Read the model definition and answer for the solid it produces. Units are mm, in the model's axes. Round coordinates to 2 decimals unless told otherwise and drop trailing zeros. Loops run counter-clockwise (first coordinate to the right, second up) from the corner with the lowest first, then second, coordinate; pieces in that order, holes last. Notation, with made-up numbers: M 15,84 L 67,84 A34 ccw 67,116 Z; hole C 48.25,29 d10. An arc over 180 degrees is marked long. Write each question's results on one line, items separated by ' | '.
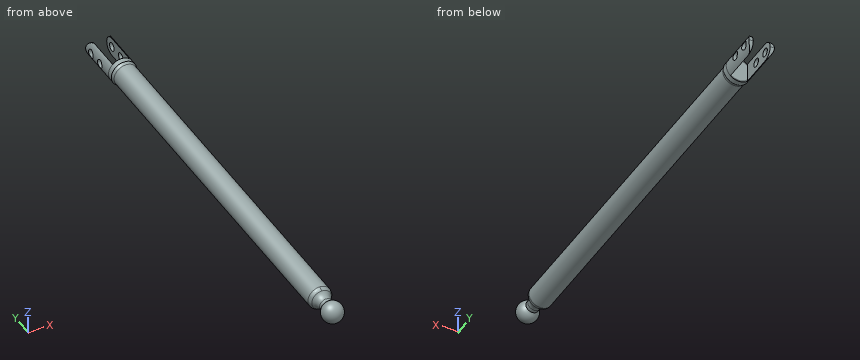
from build123d import *

# Parameters (mm, degrees)
ESBO_O2_R                         = 6
RESSALTO_EXTRUS_O1_DEPTH          = 20
ESBO_O3_R                         = 11
RESSALTO_EXTRUS_O2_DEPTH          = 350
FILETE1_R                         = 10
FILETE2_R                         = 5
RESSALTO_EXTRUS_O3_DEPTH          = 40
RESSALTO_EXTRUS_O4_START          = -5
ESBO_O7_R                         = 12
RESSALTO_EXTRUS_O4_DEPTH          = 5
FILETE3_R                         = 5
CORTE_EXTRUS_O1_DEPTH             = 17.5
CORTE_EXTRUS_O2_REACH             = 412.663
ESBO_O10_R                        = 4
CORTE_EXTRUS_O2_DIRECTION_2_REACH = 412.663


with BuildPart() as part:
    # Esboço1 → Revolução1 (revolve)
    with BuildSketch(Plane.XY):
        with BuildLine():
            Line((-10, 0), (10, 0))
            ThreePointArc((10, 0), (0, 10), (-10, 0))
        make_face()
    revolve(axis=Axis((-10, 0, 0), (1, 0, 0)))

    # Esboço2 → Ressalto-extrusão1 (add)
    with BuildSketch(Plane(origin=(0, 0, 0), x_dir=(1, 0, 0), z_dir=(0, 1, 0))):
        with Locations(Location((0, 0, 0), (0, 0, 90))):
            Circle(ESBO_O2_R)
    extrude(amount=RESSALTO_EXTRUS_O1_DEPTH)

    # Esboço3 → Ressalto-extrusão2 (add)
    with BuildSketch(Plane(origin=(0, 20, 0), x_dir=(1, 0, 0), z_dir=(0, 1, 0))):
        with Locations(Location((0, 0, 0), (0, 0, 270))):
            Circle(ESBO_O3_R)
    extrude(amount=RESSALTO_EXTRUS_O2_DEPTH)

    # Filete1
    # the kernel refuses this fillet: 10 mm, written as the material it adds along each edge
    with BuildSketch(Plane(origin=(0, 20, 0), x_dir=(0, 0, -1), z_dir=(1, 0, 0))) as filete1_piece_1:
        with BuildLine():
            CenterArc((16, -8.660254038), FILETE1_R, 120, 60)
            Line((6, -8.660254038), (5.8, -8.660254038))
            Line((5.8, -8.660254038), (5.8, 0))
            Line((5.8, 0), (6, 0.2))
            ThreePointArc((6, 0.2), (8.5, 0.2), (10.9, 0.173205081))
            Line((10.9, 0.173205081), (11, 0))
        make_face()
    revolve(axis=Axis((0, 20, 0), (0, 1, 0)))

    # Filete2
    filete2_edges = [part.edges().sort_by_distance(p)[0] for p in [
        (11, 20, 0),
    ]]
    fillet(filete2_edges, radius=FILETE2_R)

    # Esboço5 → Ressalto-extrusão3 (add)
    with BuildSketch(Plane(origin=(0, 370, 0), x_dir=(1, 0, 0), z_dir=(0, 1, 0))):
        with BuildLine():
            Line((-8, -8.94427191), (-8, 8.94427191))
            ThreePointArc((-8, 8.94427191), (-12, 0), (-8, -8.94427191))
        make_face()
        with BuildLine():
            Line((8, -8.94427191), (8, 8.94427191))
            ThreePointArc((8, 8.94427191), (12, 0), (8, -8.94427191))
        make_face()
    extrude(amount=RESSALTO_EXTRUS_O3_DEPTH)

    # Esboço7 → Ressalto-extrusão4 (add)
    with BuildSketch(Plane(origin=(0, 370, 0), x_dir=(1, 0, 0), z_dir=(0, 1, 0)).offset(RESSALTO_EXTRUS_O4_START)):
        with Locations(Location((0, 0, 0), (0, 0, 131.810314896))):
            Circle(ESBO_O7_R)
    extrude(amount=RESSALTO_EXTRUS_O4_DEPTH)

    # Filete3
    # the kernel refuses this fillet: 5 mm, written as the material it adds along each edge
    with BuildSketch(Plane(origin=(0, 365, 0), x_dir=(0, 0, 1), z_dir=(1, 0, 0))) as filete3_piece_1:
        with BuildLine():
            CenterArc((16, 3), FILETE3_R, 180, 36.869897646)
            Line((12, 0), (11.92, -0.06))
            ThreePointArc((11.92, -0.06), (11.5, -0.1), (11, -0.1))
            Line((11, -0.1), (10.9, 0))
            Line((10.9, 0), (10.9, 3))
            Line((10.9, 3), (11, 3))
        make_face()
    revolve(axis=Axis((0, 365, 0), (0, -1, 0)))

    # Esboço9 → Corte-extrusão1 (cut, symmetric)
    with BuildSketch(Plane(origin=(0, 0, 0), x_dir=(0, 0, -1), z_dir=(1, 0, 0))):
        with BuildLine():
            Line((-8.94427191, 410), (-8.94427191, 401.05572809))
            ThreePointArc((-8.94427191, 401.05572809), (-6.32455539, 407.38028334), (-1.98e-07, 410))
            Line((-1.98e-07, 410), (-8.94427191, 410))
        make_face()
        with BuildLine():
            Line((8.94427191, 410), (-1.98e-07, 410))
            ThreePointArc((-1.98e-07, 410), (6.32455525, 407.38028348), (8.94427191, 401.05572809))
            Line((8.94427191, 401.05572809), (8.94427191, 410))
        make_face()
    extrude(amount=CORTE_EXTRUS_O1_DEPTH, both=True, mode=Mode.SUBTRACT)

    # Esboço10 → Corte-extrusão2 (cut, up to next)
    with BuildSketch(Plane.ZY.offset(-8), mode=Mode.PRIVATE) as corte_extrus_o2_sk1:
        with Locations((0, 385.527864045)):
            Circle(ESBO_O10_R)
    corte_extrus_o2_tool1 = extrude(corte_extrus_o2_sk1.sketch, amount=-CORTE_EXTRUS_O2_REACH, mode=Mode.PRIVATE) & part.part
    # Esboço10 → Corte-extrusão2 (cut, up to next)
    with BuildSketch(Plane.ZY.offset(-8), mode=Mode.PRIVATE) as corte_extrus_o2_sk2:
        with Locations((0, 401.05572809)):
            Circle(ESBO_O10_R)
    corte_extrus_o2_tool2 = extrude(corte_extrus_o2_sk2.sketch, amount=-CORTE_EXTRUS_O2_REACH, mode=Mode.PRIVATE) & part.part
    add(corte_extrus_o2_tool1.solids().sort_by_distance((8, 385.527864, 0))[0], mode=Mode.SUBTRACT)
    add(corte_extrus_o2_tool2.solids().sort_by_distance((8, 401.055728, 0))[0], mode=Mode.SUBTRACT)

    # Esboço10 → Corte-extrusão2 direction 2 (cut, up to next)
    with BuildSketch(Plane.ZY.offset(-8), mode=Mode.PRIVATE) as corte_extrus_o2_direction_2_sk1:
        with Locations((0, 385.527864045)):
            Circle(ESBO_O10_R)
    corte_extrus_o2_direction_2_tool1 = extrude(corte_extrus_o2_direction_2_sk1.sketch, amount=CORTE_EXTRUS_O2_DIRECTION_2_REACH, mode=Mode.PRIVATE) & part.part
    # Esboço10 → Corte-extrusão2 direction 2 (cut, up to next)
    with BuildSketch(Plane.ZY.offset(-8), mode=Mode.PRIVATE) as corte_extrus_o2_direction_2_sk2:
        with Locations((0, 401.05572809)):
            Circle(ESBO_O10_R)
    corte_extrus_o2_direction_2_tool2 = extrude(corte_extrus_o2_direction_2_sk2.sketch, amount=CORTE_EXTRUS_O2_DIRECTION_2_REACH, mode=Mode.PRIVATE) & part.part
    add(corte_extrus_o2_direction_2_tool1.solids().sort_by_distance((8, 385.527864, 0))[0], mode=Mode.SUBTRACT)
    add(corte_extrus_o2_direction_2_tool2.solids().sort_by_distance((8, 401.055728, 0))[0], mode=Mode.SUBTRACT)


solid = part.part
Item 1: Flat-ended cylindrical pins translate along their axes: pin 1 (6 mm diameter, centred on y = 177.5, z = -7.5, fed in from +X); pin 2 (3 mm diameter, centred on x = -8, y = 226, fed in from +Z); pin 3 (1.3 mm diameter, centred on x = 1.5, z = -9.5, fed in from +Y); pin 4 (6.5 mm diameter, centred on y = 401.06, z = 0, fed in from +X). Find the tip coordinate at first contact, or state that the pin passes through.
Outcome:
pin 1: stops at x = 10.04 | pin 2: stops at z = 8.87 | pin 3: stops at y = 370 | pin 4: passes through
Item 2: Straight lines are drawn through the part: line 1 (Y direction, x = -10.25, z = 2); line 2 (X direction, y = 107, z = -0.5); line 3 (Y direction, x = 2.25, z = 3.75). For each, find the intervals that lie inside material, in ascending order.
Outcome:
line 1: y = 20.23 to 382.06, 388.99 to 397.59, 404.52 to 409.77 | line 2: x = -10.99 to 10.99 | line 3: y = -8.99 to 370
Item 3: The part is cut by section A-A (y = 105). Determine the outline of the cut face in (x, z).
Outcome:
outline: C 0,0 d22
